Model file for the job. Use its own axes, mm. Face numbers are marked on the shaded views. A direction names the side the tool comes from. Round coordinates to 2 decimals unless told otherwise and drop trailing zeros. Loops run counter-clockwise (first coordinate to the right, second up) from the corner with the lowest first, then second, coordinate; pieces in that order, holes last. Notation, with made-up numbers: M 71,16.25 L 123,16.25 A17 ccw 123,44.25 Z; hole C 16.25,-20 d11. An arc over 180 degrees is marked long. Use a Markdown table: item, result. Add a question column.
Item 1: Tool access for the marked faces 1 and 2: list every direction of +Z, -Z, +X, -X, +Y, -Y with a clear straight run to the whole face (end or side of a thin tool).
Item 2: Pin check, flat tips, straight feed: P1, Ø2, axis at x = 2, y = 0, coming from the -Z side; P2, Ø1, axis at x = -0.5, z = 8, coming from the -Y side; P3, Ø2, axis at x = -1.5, z = 11.5, coming from the -Y side. Stop position of each tip, or through.
Item 3: Wall check: L1, parallel to Y at x = 0, z = 22; L2, parallel to Y at x = 0.75, z = 29.5; L3, parallel to Y at x = 1.25, z = 29.5. Give the ranges that are in metal, low to high. Write a range as from..to.
Item 4: Saw through at A-A on z = 6.5. Write the cut outline in (x, y), then the cut area to 3 significant figures.
```python
from build123d import *

# Parameters (mm, degrees)
F3_DEPTH = 0.8
F3_TAPER = 30


with BuildPart() as f1:
    # F0 (on Front) → F1 (revolve)
    with BuildSketch(Plane.XZ):
        Polygon((0, 30), (0, 0), (1.5, 1.5), (1.5, 28), (3.5, 30), align=None)
    revolve(axis=Axis((0, 0, 15), (0, 0, 1)))

    # F2 (on face) → F3 (cut)
    with BuildSketch(Plane.XY.offset(30)):
        Polygon((0.5, 2.5), (-0.5, 2.5), (-0.5, 0.5), (-2.5, 0.5), (-2.5, -0.5), (-0.5, -0.5), (-0.5, -2.5), (0.5, -2.5), (0.5, -0.5), (2.5, -0.5), (2.5, 0.5), (0.5, 0.5), align=None)
    extrude(amount=-F3_DEPTH, taper=F3_TAPER, mode=Mode.SUBTRACT)


solid = f1.part
```
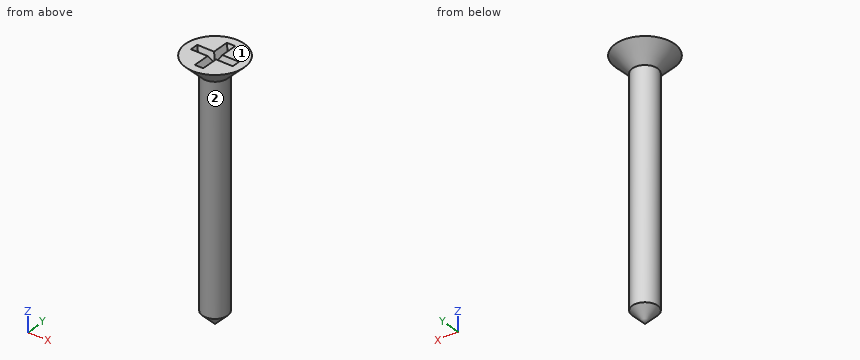
Entries:
| question | item | result |
|---|---|---|
| 1 | face 1 | +Z, +X, -X, +Y, -Y |
| 1 | face 2 | -Z |
| 2 | P1 | z = 1 |
| 2 | P2 | y = -1.5 |
| 2 | P3 | y = -1.41 |
| 3 | L1 | -1.5..1.5 |
| 3 | L2 | -2.9..-0.21, 0.21..2.9 |
| 3 | L3 | -2.73..-0.21, 0.21..2.73 |
| 4 | outline | C 0,0 d3 |
| 4 | area | 7.07 mm2 |
